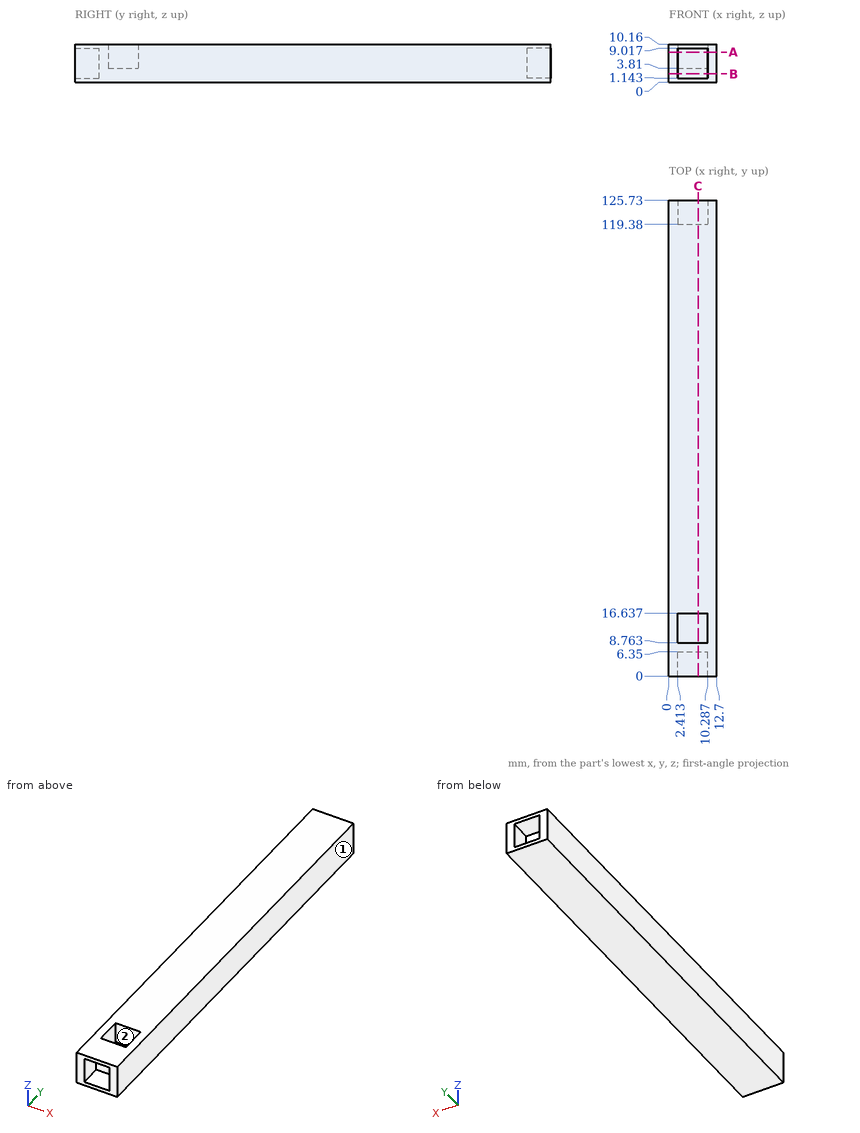
Verification items for this drawing (mm, ordinates from the low corner). Round coordinates to 2 decimals unless told otherwise and drop trailing zeros. Order: outer loops, then holes, each group sorted by start corner. A loop starts at its lowest first (then second) coordinate and runs counter-clockwise, first axis right, second up. Notation, with made-up numbers: (53.5, 77) - (68.5, 77) arc R19 cw to (68.5, 91) - close; hole circle Ø8 at (89.25, 3). An arc over 180 degrees is marked (long way). Use CSV: the item, a comma, the result in double quotes.
(1) Thickness scan on probe 1 along Y at (x, z) = (4.75, 5.25); probe 2 along X at (y, z) = (6, 8); probe 3 along Y at (x, z) = (9, 3.25). Record the ranges inside material, lowest first. Write a range as from..to.
Entries:
probe 1,"6.35..8.76, 16.64..119.38"
probe 2,"0..2.41, 10.29..12.7"
probe 3,"6.35..119.38"
(2) Section check A-A on z = 8. Record the boundary of the cut face in (x, y), and give its area (3 significant figures).
Entries:
outline,"(0, 0) - (2.41, 0) - (2.41, 6.35) - (10.29, 6.35) - (10.29, 0) - (12.7, 0) - (12.7, 125.73) - (10.29, 125.73) - (10.29, 119.38) - (2.41, 119.38) - (2.41, 125.73) - (0, 125.73) - close; hole (2.41, 8.76) - (10.29, 8.76) - (10.29, 16.64) - (2.41, 16.64) - close"
area,"1,430 mm^2"
(3) Mould release check, pull along Y, two halves, no side actions. Record for the marked faces 1 and 2: released by +Y, released by -Y, zero draft, split by the parting line, or undercut.
Entries:
face 1,"zero draft"
face 2,"undercut"
(4) Section check C-C on x = 7.75. Record the boundary of the cut face in (y, z).
Entries:
outline,"(0, 0) - (125.73, 0) - (125.73, 1.14) - (119.38, 1.14) - (119.38, 9.02) - (125.73, 9.02) - (125.73, 10.16) - (16.64, 10.16) - (16.64, 3.81) - (8.76, 3.81) - (8.76, 10.16) - (0, 10.16) - (0, 9.02) - (6.35, 9.02) - (6.35, 1.14) - (0, 1.14) - close"
(5) Gauge pin test, flat end, axial feed: pin 1 Ø1.9 at (x, z) = (8, 7) entering from +Y. Record the tip position at first contact, or that the pin passes through.
Entries:
pin 1,"y = 119.38"
(6) Section check B-B on z = 2.25. Record the boundary of the cut face in (x, y), and give its area (3 significant figures).
Entries:
outline,"(0, 0) - (2.41, 0) - (2.41, 6.35) - (10.29, 6.35) - (10.29, 0) - (12.7, 0) - (12.7, 125.73) - (10.29, 125.73) - (10.29, 119.38) - (2.41, 119.38) - (2.41, 125.73) - (0, 125.73) - close"
area,"1,500 mm^2"
